from build123d import *

# Parameters (mm, degrees)
SKETCH1_W           = 52
SKETCH1_H           = 2.6
BOSS_EXTRUDE1_DEPTH = 2.5
SKETCH2_R           = 1.55
CUT_EXTRUDE1_DEPTH  = 10


with BuildPart() as part:
    # Sketch1 → Boss-Extrude1 (new body)
    with BuildSketch(Plane(origin=(0, 0, 0), x_dir=(1, 0, 0), z_dir=(0, 1, 0))):
        Polygon((72, -25), (76, -25), (76, 25), (72, 25), (72, 72.1), (-72, 72.1), (-72, 25), (-76, 25), (-76, -25), (-72, -25), (-72, -72.1), (72, -72.1), align=None)
        with Locations((0, -67.8)):
            Rectangle(SKETCH1_W, SKETCH1_H, mode=Mode.SUBTRACT)
        with Locations((0, 67.8)):
            Rectangle(SKETCH1_W, SKETCH1_H, mode=Mode.SUBTRACT)
    extrude(amount=BOSS_EXTRUDE1_DEPTH)

    # Sketch2 → Cut-Extrude1 (cut)
    with BuildSketch(Plane(origin=(0, 2.5, 0), x_dir=(1, 0, 0), z_dir=(0, 1, 0))):
        with Locations((-42.5, 52.1)):
            Circle(SKETCH2_R)
        with Locations((42.5, 52.1)):
            Circle(SKETCH2_R)
    extrude(amount=-CUT_EXTRUDE1_DEPTH, mode=Mode.SUBTRACT)


solid = part.part
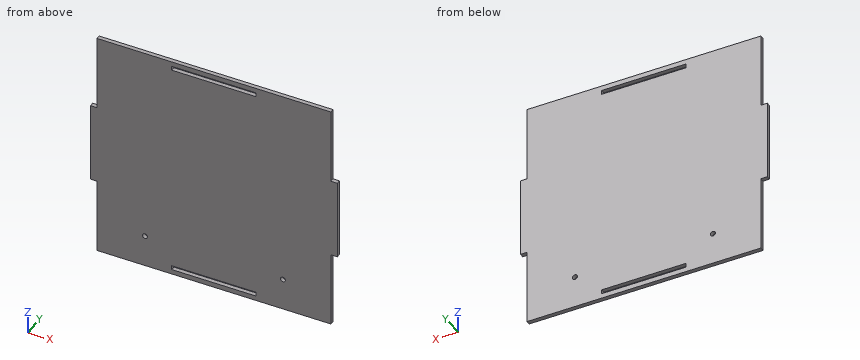
The listing builds one solid part. Answer for the finished solid, in the listing's coordinates (mm). Round coordinates to 2 decimals unless told otherwise and drop trailing zeros. Order: outer loops, then holes, each group sorted by start corner. A loop starts at its lowest first (then second) coordinate and runs counter-clockwise, first axis right, second up. Notation, with made-up numbers: M 79,53 L 99,53 A8 cw 99,62 Z; hole C -3,-34 d1. An arc over 180 degrees is marked long. Answer in a Markdown table with one row per item. Add a question column.
1) Flat-ended cylindrical pins translate along their axes: pin 1 Ø1.2 at (x, y) = (-73.5, 1) entering from +Z; pin 2 Ø1.2 at (y, z) = (1, 67.5) entering from -X; pin 3 Ø2.5 at (x, z) = (-42.5, -52.1) entering from +Y; pin 4 Ø1.2 at (y, z) = (1, -47.5) entering from +X. Find the tip coordinate at first contact, or state that the pin passes through.
2) Consider line 1 along X through (y, z) = (1.15, -52.1); line 2 along Z through (x, y) = (12, 2.2); line 3 along Z through (x, y) = (42.5, 0.8). Determine where each line is inside the solid, lowest interval first. Write a range as from..to.
3) The part is cut by section B-B on x = -9.5. Determine the outline of the cut face in (y, z).
4) The part is cut by section A-A on y = 2.1. Determine the outline of the cut face in (x, z).
5) The part is cut by section C-C on z = -32. Determine the outline of the cut face in (x, y), plus the area to 3 significant figures.
Findings below:
| question | item | result |
|---|---|---|
| 1 | pin 1 | stops at z = 25 |
| 1 | pin 2 | stops at x = -72 |
| 1 | pin 3 | passes through |
| 1 | pin 4 | stops at x = 72 |
| 2 | line 1 | x = -72..-44.05, -40.95..40.95, 44.05..72 |
| 2 | line 2 | z = -72.1..-69.1, -66.5..66.5, 69.1..72.1 |
| 2 | line 3 | z = -72.1..-53.65, -50.55..72.1 |
| 3 | outline | M 0,-72.1 L 2.5,-72.1 L 2.5,-69.1 L 0,-69.1 Z; M 0,-66.5 L 2.5,-66.5 L 2.5,66.5 L 0,66.5 Z; M 0,69.1 L 2.5,69.1 L 2.5,72.1 L 0,72.1 Z |
| 4 | outline | M -76,-25 L -72,-25 L -72,-72.1 L 72,-72.1 L 72,-25 L 76,-25 L 76,25 L 72,25 L 72,72.1 L -72,72.1 L -72,25 L -76,25 Z; hole C -42.5,-52.1 d3.1; hole M -26,-69.1 L 26,-69.1 L 26,-66.5 L -26,-66.5 Z; hole M -26,66.5 L 26,66.5 L 26,69.1 L -26,69.1 Z; hole C 42.5,-52.1 d3.1 |
| 5 | outline | M -72,0 L 72,0 L 72,2.5 L -72,2.5 Z |
| 5 | area | 360 mm² |
